from build123d import *

# Parameters (mm, degrees)
EXTRUDE_2_DEPTH     = 16
SKETCH_3_W          = 12
SKETCH_3_H          = 12
CUT_EXTRUDE_3_DEPTH = 25
SKETCH_6_W          = 6
SKETCH_6_H          = 15
CUT_EXTRUDE_4_DEPTH = 25


with BuildPart() as part:
    # 스케치1 → 보스-돌출2 (new body)
    with BuildSketch(Plane.XY):
        Polygon((31.5, 0), (-31.5, 0), (-16.5, 5), (-11.5, 10), (-8.457539251, 30), (8.457539251, 30), (11.5, 10), (16.5, 5), align=None)
    extrude(amount=EXTRUDE_2_DEPTH)

    # 스케치3 → 컷-돌출3 (cut)
    with BuildSketch(Plane(origin=(0, 30, 0), x_dir=(1, 0, 0), z_dir=(0, 1, 0))):
        with Locations((0, -8)):
            Rectangle(SKETCH_3_W, SKETCH_3_H)
    extrude(amount=-CUT_EXTRUDE_3_DEPTH, mode=Mode.SUBTRACT)

    # 스케치6 → 컷-돌출4 (cut)
    with BuildSketch(Plane.XY.offset(16)):
        with Locations((3, 22.5)):
            Rectangle(SKETCH_6_W, SKETCH_6_H)
        with Locations((-3, 22.5)):
            Rectangle(SKETCH_6_W, SKETCH_6_H)
    extrude(amount=-CUT_EXTRUDE_4_DEPTH, mode=Mode.SUBTRACT)


solid = part.part
Can you work these out from the model? Positions are in its coordinate system, mm. A direction names the side the tool comes from. Give positions to 0.01 mm unless a question says otherwise; leave off trailing zeros. Write each loop counter-clockwise with the first axis right and the second up, starting at its lowest first coordinate (ties: lowest second). Pieces come first, ordered by that corner, then holes. Notation, with made-up numbers: (68.5, 23.5) -> (80.5, 23.5) arc R9 cw to (80.5, 32.5) -> close; hole circle Ø9 at (35, -30). An arc over 180 degrees is marked (long way). Answer as a JSON object with one key per item and string values. Group by question number.
Item 1: For faces 1 (the face through (0, 15, 1)), 2 (the face through (0, 0, 8)), 3 (the face through (0, 10, 2)), which set-ups out of +Z, -Z, +X, -X, +Y, -Y let a thin tool reach every point of the face, with its end or its side?
Item 2: I'm going to push flat-ended pins straight in: P1, Ø8, axis at x = 25, z = 3.5, coming from the +Y side; P2, Ø6, axis at x = -22, z = 7, coming from the +Y side; P3, Ø2, axis at x = 2.5, z = 0.5, coming from the +Y side; P4, Ø10, axis at x = 19.5, y = 17.5, coming from the +Z side. Where does each tip first touch, or does it pass through?
Item 3: Suppose I cut it at C-C (y = 24.25). Please give me the cut outline in (x, z), plus the area to 3 significant figures.
Item 4: Suppose I cut it at B-B (z = 12.5). Please give me the cut outline in (x, y).
Item 5: Suppose I cut it at D-D (x = -2.5). Please give me the cut outline in (y, z), plus the area to 3 significant figures.
Item 6: Please list where these lines run through material, in increasing order: line 1 (Z direction, x = 5.5, y = 10.75); line 2 (X direction, y = 25, z = 11); line 3 (X direction, y = 22.25, z = 2.5). Write a range as [from, to].
Item 7: We'd pull the mould along X, two halves only. Please class faces 4 (the face through (14, 7.5, 7.9)), 5 (the face through (0, 15, 15)), 6 (the face through (7, 30, 8)): +X half, -X half, draft (parallel to the pull), parting line (faces both ways), or undercut.
Item 8: Suppose I cut it at A-A (y = 5.75). Please give me the cut outline in (x, z).
Findings:
{
 "1": {"face 1": "+Z, -Z, +Y", "face 2": "+Z, -Z, +X, -X, -Y", "face 3": "+Y"},
 "2": {"P1": "stops at y = 3.5", "P2": "stops at y = 4.17", "P3": "stops at y = 15", "P4": "passes through"},
 "3": {"outline": "(-9.33, 0) -> (-6, 0) -> (-6, 16) -> (-9.33, 16) -> close; (6, 0) -> (9.33, 0) -> (9.33, 16) -> (6, 16) -> close", "area": "107 mm²"},
 "4": {"outline": "(-31.5, 0) -> (31.5, 0) -> (16.5, 5) -> (11.5, 10) -> (8.46, 30) -> (6, 30) -> (6, 5) -> (-6, 5) -> (-6, 30) -> (-8.46, 30) -> (-11.5, 10) -> (-16.5, 5) -> close"},
 "5": {"outline": "(0, 0) -> (15, 0) -> (15, 2) -> (5, 2) -> (5, 14) -> (15, 14) -> (15, 16) -> (0, 16) -> close", "area": "120 mm²"},
 "6": {"line 1": "z = [0, 2], [14, 16]", "line 2": "x = [-9.22, -6], [6, 9.22]", "line 3": "x = [-9.64, -6], [6, 9.64]"},
 "7": {"face 4": "+X half", "face 5": "undercut", "face 6": "draft"},
 "8": {"outline": "(-15.75, 0) -> (15.75, 0) -> (15.75, 16) -> (-15.75, 16) -> close; hole (-6, 2) -> (6, 2) -> (6, 14) -> (-6, 14) -> close"}
}
